```python
from build123d import *

# Parameters (mm, degrees)
F0_R     = 5.925
F1_DEPTH = 31.7
F2_R     = 4.865
F3_DEPTH = 21.6
F4_R     = 5.925
F4_R_2   = 4.865
F5_DEPTH = 26.7
F7_D     = 4.26
F8_SIZE  = 0.05
F9_SIZE  = 0.05


with BuildPart() as f1:
    # F0 (on Right) → F1 (new body)
    with BuildSketch(Plane.YZ):
        Circle(F0_R)
    extrude(amount=F1_DEPTH)

    # F2 (on face) → F3 (join)
    with BuildSketch(Plane.YZ.offset(31.7)):
        Circle(F2_R)
    extrude(amount=F3_DEPTH)

    # F4 (on face) → F5 (join)
    with BuildSketch(Plane.YZ.offset(53.3)):
        Circle(F4_R)
        Circle(F4_R_2, mode=Mode.SUBTRACT)
        Circle(F4_R_2)
    extrude(amount=F5_DEPTH)

    # F7 (through all)
    with Locations(Plane.YZ.offset(80)):
        with Locations((0, 0)):
            Hole(F7_D / 2)

    # F8
    f8_edges = [f1.edges().sort_by_distance(p)[0] for p in [
        (31.7, -5.925, 0),
    ]]
    chamfer(f8_edges, length=F8_SIZE)

    # F9
    f9_edges = [f1.edges().sort_by_distance(p)[0] for p in [
        (53.3, -5.925, 0),
    ]]
    chamfer(f9_edges, length=F9_SIZE)


solid = f1.part
```
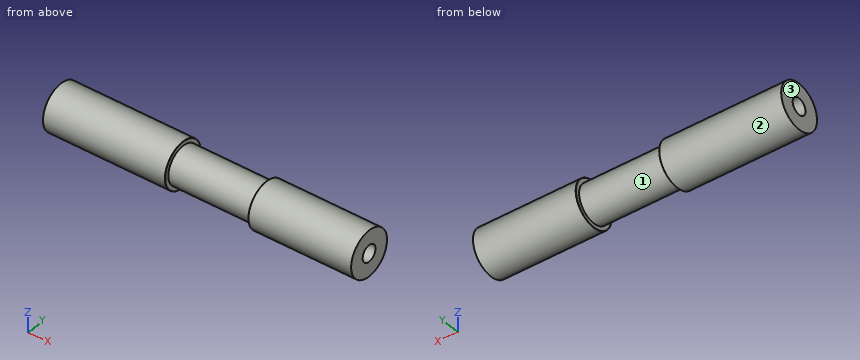
CAD build for the part. Positions are in the model's coordinates, mm. Face numbers are marked on the shaded views. Coordinates: 2 decimals unless noted, no trailing zeros. Order: outer loops, then holes, each group sorted by start corner. A loop starts at its lowest first (then second) coordinate and runs counter-clockwise, first axis right, second up. Notation, with made-up numbers: (0, -6) - (46, -6) arc R29 ccw to (46, 22) - close; hole circle Ø11 at (36.25, 50.5). An arc over 180 degrees is marked (long way). Use a Markdown table: item, result. Add a question column.
(1) Flat gauge pins, fed straight in: pin 1 (1.5 mm diameter, centred on x = 44, z = -3, fed in from -Y); pin 2 (1.5 mm diameter, centred on x = 56.5, z = -1.5, fed in from -Y); pin 3 (2 mm diameter, centred on x = 9, y = -2.5, fed in from +Z). Where does each tip first touch, or does it go through?
(2) Saw through at C-C (x = 22.5). Give the cut face in (y, z) (3 decimals), then the cut area to 3 significant figures.
(3) Drill centre lines: line 1 along Z through (x, y) = (59, 0) (3 decimals); line 2 along Z through (x, y) = (51.5, 0) (3 decimals); line 3 along Y through (x, z) = (12, -1.75). Where is each one in solid material? Low to high. Write a range as [from, to].
(4) Saw through at A-A (y = 0). Give the cut face in (x, z) (3 decimals).
(5) Saw through at D-D (x = 34). Give the cut face in (y, z) (3 decimals), then the cut area to 3 significant figures.
(6) Pull direction X, two halves, no side cores. Call the marked faces 1, 2 and 3: +X half, -X half, draft (parallel to the pull), parting line (faces both ways), or undercut.
Solved:
| question | item | result |
|---|---|---|
| 1 | pin 1 | stops at y = -4.31 |
| 1 | pin 2 | stops at y = -5.88 |
| 1 | pin 3 | stops at z = 5.73 |
| 2 | outline | circle Ø11.85 at (0, 0); hole circle Ø4.26 at (0, 0) |
| 2 | area | 96.0 mm² |
| 3 | line 1 | z = [-5.925, -2.13], [2.13, 5.925] |
| 3 | line 2 | z = [-4.865, -2.13], [2.13, 4.865] |
| 3 | line 3 | y = [-5.66, -1.21], [1.21, 5.66] |
| 4 | outline | (0, -5.925) - (31.65, -5.925) - (31.7, -5.875) - (31.7, -4.865) - (53.3, -4.865) - (53.3, -5.875) - (53.35, -5.925) - (80, -5.925) - (80, -2.13) - (0, -2.13) - close; (0, 2.13) - (80, 2.13) - (80, 5.925) - (53.35, 5.925) - (53.3, 5.875) - (53.3, 4.865) - (31.7, 4.865) - (31.7, 5.875) - (31.65, 5.925) - (0, 5.925) - close |
| 5 | outline | circle Ø9.73 at (0, 0); hole circle Ø4.26 at (0, 0) |
| 5 | area | 60.1 mm² |
| 6 | face 1 | undercut |
| 6 | face 2 | draft |
| 6 | face 3 | -X half |
